Geometry: see drawing. Coordinates: mm, zero at the bounding-box minimum. A direction names the side the tool comes from. Give positions to 0.01 mm unless a question says otherwise; leave off trailing zeros. Loops run counter-clockwise (first coordinate to the right, second up) from the corner with the lowest first, then second, coordinate; pieces in that order, holes last. Notation, with made-up numbers: M 9.25,-3.5 L 30.25,-3.5 A27 ccw 30.25,24.5 Z; hole C -19.75,30 d5. An arc over 180 degrees is marked long. Return JSON: item names as keys, results as strings. Group by question number.
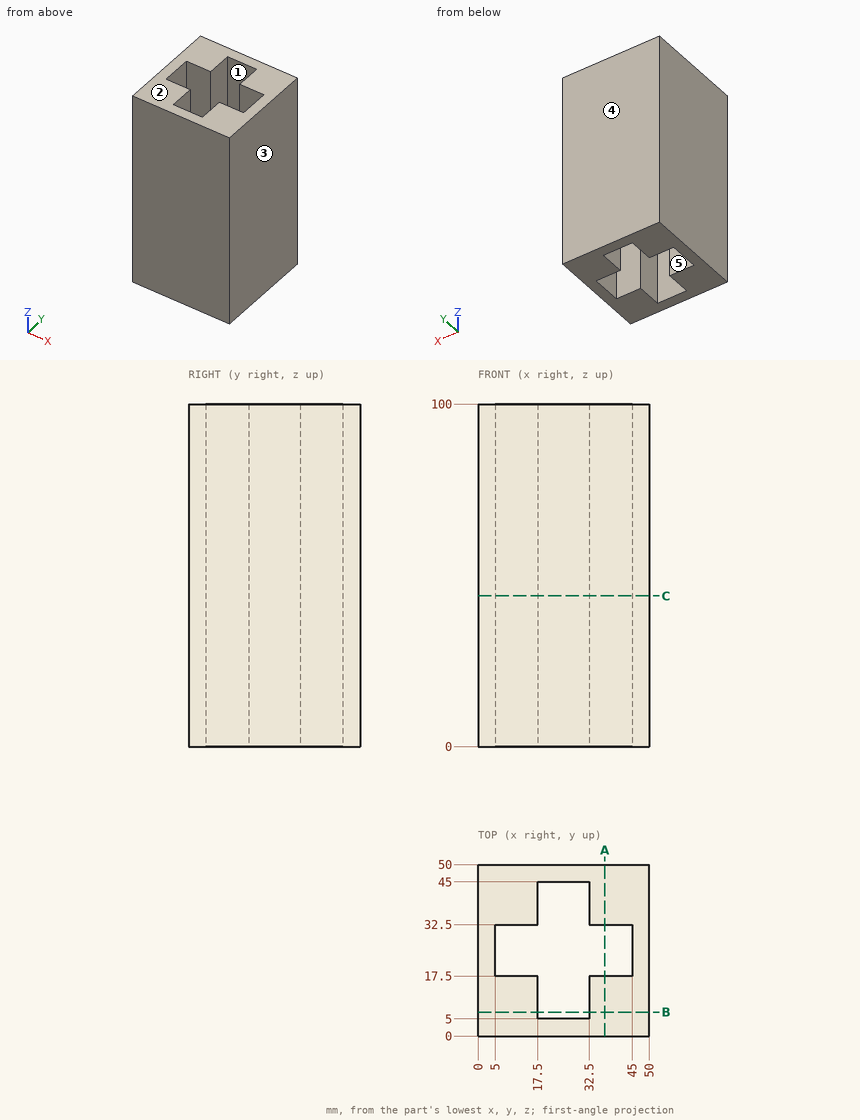
Item 1: Section C-C, the plane z = 44. Return loops of the section in (x, y).
Item 2: Section A-A, the plane x = 37. Return loops of the section in (y, z).
Item 3: Reachability of the marked faces 1 and 2 from +Z, -Z, +X, -X, +Y, -Y: full face, straight path, thin tool, end or side. Return the list, or none.
Item 4: Material intervals for line 1 (Y direction, x = 22.5, z = 21.5); line 2 (Y direction, x = 40.5, z = 11), sorted ascending. Write a range as from..to.
Item 5: Pull-direction query (X, two-part tool) for the marked faces 3, 4 and 5; classes: pulls with the +X half, pulls with the -X half, needs draft (parallel to the pull), parting line crosses it, or undercut.
Answer below:
{
 "1": {"outline": "M 0,0 L 50,0 L 50,50 L 0,50 Z; hole M 5,17.5 L 17.5,17.5 L 17.5,5 L 32.5,5 L 32.5,17.5 L 45,17.5 L 45,32.5 L 32.5,32.5 L 32.5,45 L 17.5,45 L 17.5,32.5 L 5,32.5 Z"},
 "2": {"outline": "M 0,0 L 17.5,0 L 17.5,100 L 0,100 Z; M 32.5,0 L 50,0 L 50,100 L 32.5,100 Z"},
 "3": {"face 1": "+Z, -Z", "face 2": "+Z, +X, -X, +Y, -Y"},
 "4": {"line 1": "0..5, 45..50", "line 2": "0..17.5, 32.5..50"},
 "5": {"face 3": "pulls with the +X half", "face 4": "needs draft", "face 5": "undercut"}
}
